Could you check a few things on this drawing? It's one solid part, dimensions in mm from its lowest x, y, z. Round coordinates to 2 decimals unless told otherwise and drop trailing zeros. Order: outer loops, then holes, each group sorted by start corner. A loop starts at its lowest first (then second) coordinate and runs counter-clockwise, first axis right, second up. Notation, with made-up numbers: M 39.25,83.5 L 44.25,83.5 A25 ccw 44.25,104.5 Z; hole C 52,79 d4. An arc over 180 degrees is marked long. Answer as a JSON object with one key per item and string values. Group by question number.
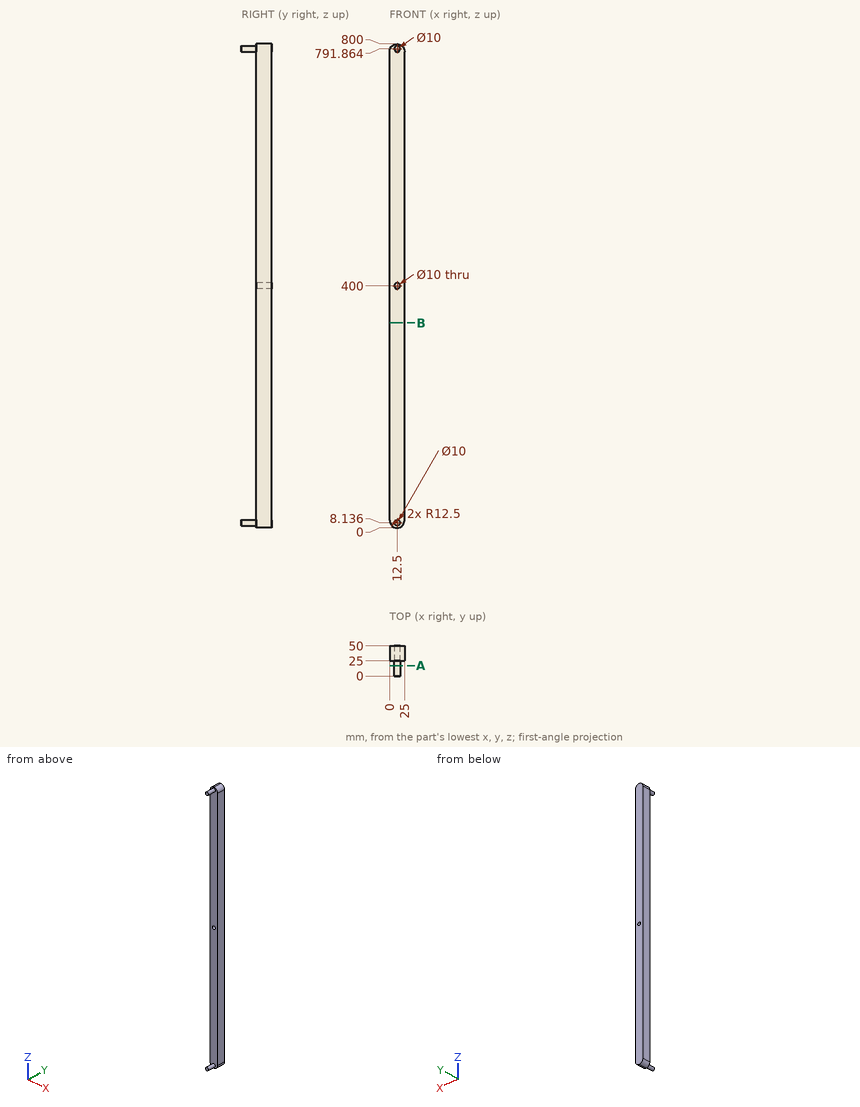
1) If we section it at B-B on z = 339: Write out the boundary of the cut face in (x, y).
2) For pin 1 (5 mm diameter, centred on x = 11, y = 12, fed in from -Z); pin 2 (1.5 mm diameter, centred on x = 3.5, z = 624, fed in from -Y); pin 3 (8 mm diameter, centred on y = 18.5, z = 122, fed in from -X), each with a flat end and sliding along its axis, tell me the tip position at first contact or that it passes through.
3) I need wall thicknesses on line 1 along X through (y, z) = (40.5, 400); line 2 along Z through (x, y) = (11.25, 26.5); line 3 along Y through (x, z) = (16.25, 705). Which ranges of each line are inside material? Lowest first, please.
4) If we section it at A-A on y = 17: Write out the boundary of the cut face in (x, z).
Findings:
{
 "1": {"outline": "M 0,25 L 25,25 L 25,50 L 0,50 Z"},
 "2": {"pin 1": "stops at z = 3.14", "pin 2": "stops at y = 25", "pin 3": "passes through"},
 "3": {"line 1": "x = 0 to 7.5, 17.5 to 25", "line 2": "z = 0.06 to 395.16, 404.84 to 799.94", "line 3": "y = 25 to 50"},
 "4": {"outline": "C 12.5,8.14 d10; C 12.5,791.86 d10"}
}
